Could you check a few things on this drawing? It's one solid part, dimensions in mm from its lowest x, y, z. A direction names the side the tool comes from. Round coordinates to 2 decimals unless told otherwise and drop trailing zeros. Write each loop counter-clockwise with the first axis right and the second up, starting at its lowest first coordinate (ties: lowest second). Pieces come first, ordered by that corner, then holes. Notation, with made-up numbers: (84.5, 51.5) -> (116.5, 51.5) arc R16 ccw to (116.5, 63.5) -> close; hole circle Ø10 at (42.25, 74.5). An arc over 180 degrees is marked (long way). Answer in a Markdown table with one row per item.
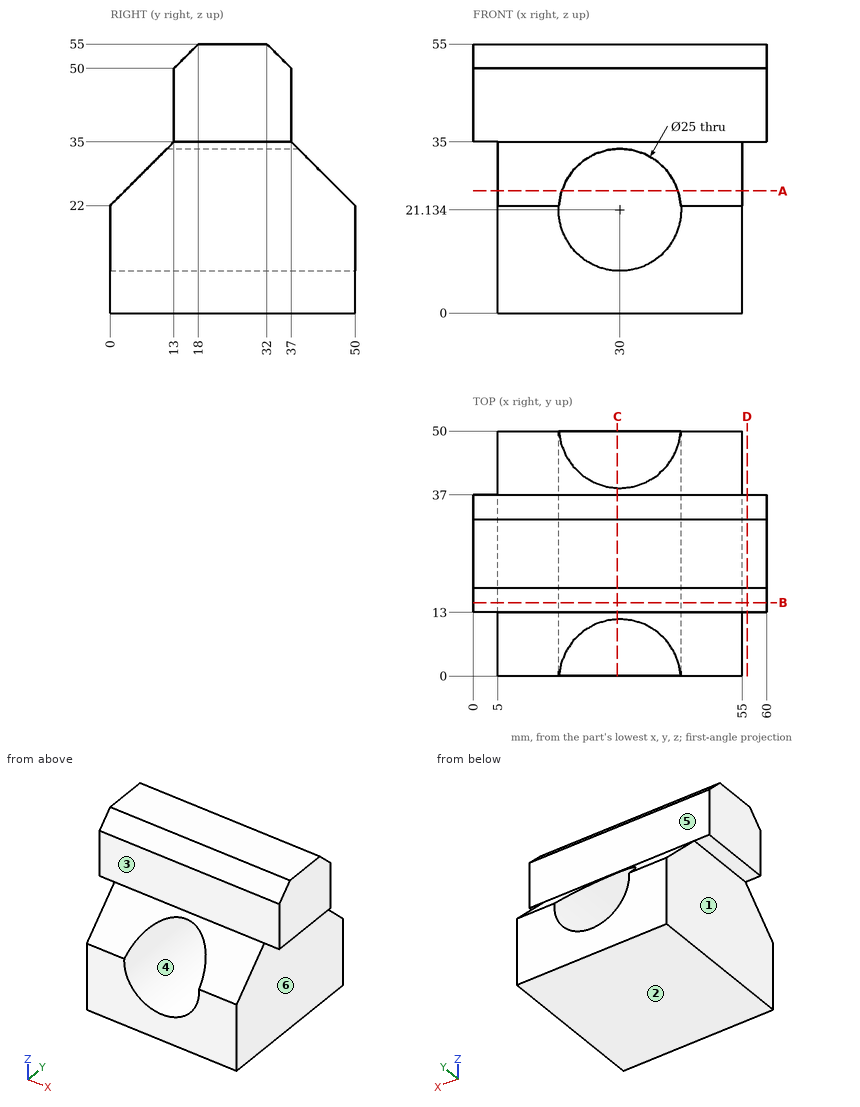
1) Imagine slicing it at C-C, the plane x = 29.5. Please give me the cut outline in (y, z), plus the area to 3 significant figures.
Findings:
| item | result |
|---|---|
| outline | (0, 0) -> (50, 0) -> (50, 8.64) -> (0, 8.64) -> close; (11.62, 33.62) -> (38.38, 33.62) -> (37, 35) -> (37, 50) -> (32, 55) -> (18, 55) -> (13, 50) -> (13, 35) -> close |
| area | 922 mm^2 |
2) For pin 1 (12 mm diameter, centred on x = 42.5, z = 43, fed in from -Y); pin 2 (12 mm diameter, centred on x = 20, z = 45.5, fed in from +Y); pin 3 (5.5 mm diameter, centred on x = 1.5, y = 21.5, fed in from -Z), each with a flat end and sliding along its axis, tell me the tip position at first contact or that it passes through.
Findings:
| item | result |
|---|---|
| pin 1 | stops at y = 13 |
| pin 2 | stops at y = 37 |
| pin 3 | stops at z = 35 |
3) Imagine slicing it at B-B, the plane y = 15. Please give me the cut outline in (x, z).
Findings:
| item | result |
|---|---|
| outline | (0, 35) -> (5, 35) -> (5, 0) -> (55, 0) -> (55, 35) -> (60, 35) -> (60, 52) -> (0, 52) -> close; hole circle Ø25 at (30, 21.13) |
4) Imagine slicing it at A-A, the plane z = 25. Please give me the cut outline in (x, y).
Findings:
| item | result |
|---|---|
| outline | (5, 3) -> (18.11, 3) -> (18.11, 47) -> (5, 47) -> close; (41.89, 3) -> (55, 3) -> (55, 47) -> (41.89, 47) -> close |
5) For the marked faces 1, 2 and 3, which set-ups out of +Z, -Z, +X, -X, +Y, -Y let a thin tool reach every point of the face, with its end or its side?
Findings:
| item | result |
|---|---|
| face 1 | -Z, -X, +Y, -Y |
| face 2 | -Z, +X, -X, +Y, -Y |
| face 3 | +Z, +X, -X, -Y |
6) Please list where these lines run through material, in increasing order: line 1 (Y direction, x = 45, z = 35); line 2 (X direction, y = 25, z = 17); line 3 (X direction, y = 32.5, z = 3.5).
Findings:
| item | result |
|---|---|
| line 1 | y = 13 to 37 |
| line 2 | x = 5 to 18.2, 41.8 to 55 |
| line 3 | x = 5 to 55 |
7) Imagine slicing it at D-D, the plane x = 56. Please give me the cut outline in (y, z).
Findings:
| item | result |
|---|---|
| outline | (13, 35) -> (37, 35) -> (37, 50) -> (32, 55) -> (18, 55) -> (13, 50) -> close |
8) Thinking about a two-plate mould opening in X: for the marked faces 4, 5 and 6, which applies, +X half, -X half, draft (parallel to the pull), parting line (faces both ways), or undercut?
Findings:
| item | result |
|---|---|
| face 4 | undercut |
| face 5 | draft |
| face 6 | +X half |
